Geometry: final body of the model. Coordinates: model frame, mm. A direction names the side the tool comes from. Round coordinates to 2 decimals unless told otherwise and drop trailing zeros. Loops run counter-clockwise (first coordinate to the right, second up) from the corner with the lowest first, then second, coordinate; pieces in that order, holes last. Notation, with made-up numbers: M -14,28.5 L 8,28.5 A30 ccw 8,64.5 Z; hole C 73,23 d4. An arc over 180 degrees is marked long. Write each question's results on one line, items separated by ' | '.
```python
from build123d import *

# Parameters (mm, degrees)
SZKIC1_W                       = 322
SZKIC1_H                       = 170
DODANIE_WYCI_GNI_CIE1_DEPTH    = 15
SZKIC2_R                       = 2
WYTNIJ_WYCI_GNI_CIE2_DEPTH     = 17.75
SZYK_LINIOWY1_COUNT            = 2
SZYK_LINIOWY1_PITCH            = 69.6
SZYK_LINIOWY1_COUNT_DIR2       = 2
SZYK_LINIOWY1_PITCH_DIR2       = 69.6
SZKIC5_R                       = 37.5
WYTNIJ_WYCI_GNI_CIE3_DEPTH     = 2
SZKIC7_R                       = 18.5
WYTNIJ_WYCI_GNI_CIE4_DEPTH     = 17.75
SZKIC10_R                      = 4
WYTNIJ_WYCI_GNI_CIE7_DEPTH     = 16
SZYK_LINIOWY3_COUNT            = 2
SZYK_LINIOWY3_PITCH            = 79
SZYK_LINIOWY2_COUNT            = 2
SZYK_LINIOWY2_PITCH            = 228
SZYK_LINIOWY2_COPY_1_SKETCH_R  = 2
SZYK_LINIOWY2_COPY_1_DEPTH     = 17.75
SZYK_LINIOWY2_COPY_2_SKETCH_R  = 2
SZYK_LINIOWY2_COPY_2_DEPTH     = 17.75
SZYK_LINIOWY2_COPY_3_SKETCH_R  = 2
SZYK_LINIOWY2_COPY_3_DEPTH     = 17.75
SZYK_LINIOWY2_COPY_4_SKETCH_R  = 4
SZYK_LINIOWY2_COPY_4_DEPTH     = 16
OTW_R_GWINTOWANY_M8X1_01_D     = 7
OTW_R_GWINTOWANY_M8X1_01_DEPTH = 21
OTW_R_GWINTOWANY_M8X1_01_TIP   = 2.103012167


with BuildPart() as part:
    # Szkic1 → Dodanie-wyci_gni_cie1 (new body)
    with BuildSketch(Plane.XY):
        Rectangle(SZKIC1_W, SZKIC1_H)
    extrude(amount=DODANIE_WYCI_GNI_CIE1_DEPTH)

    # Szkic2 → Wytnij-wyci_gni_cie2 (cut)
    with BuildSketch(Plane.XY.offset(15)):
        with Locations((-148.8, -71.87)):
            Circle(SZKIC2_R)
    wytnij_wyci_gni_cie2 = extrude(amount=-WYTNIJ_WYCI_GNI_CIE2_DEPTH, mode=Mode.SUBTRACT)

    # Szyk liniowy1: Wytnij-wyci_gni_cie2 2 × 2
    with Locations(*[(i * SZYK_LINIOWY1_PITCH, j * SZYK_LINIOWY1_PITCH_DIR2, 0) for i in range(SZYK_LINIOWY1_COUNT) for j in range(SZYK_LINIOWY1_COUNT_DIR2) if (i, j) != (0, 0)]):
        add(wytnij_wyci_gni_cie2, mode=Mode.SUBTRACT)

    # Szkic5 → Wytnij-wyci_gni_cie3 (cut)
    with BuildSketch(Plane(origin=(0, 0, 0), x_dir=(-1, 0, 0), z_dir=(0, 0, -1))):
        with Locations((114, -37.07)):
            Circle(SZKIC5_R)
    wytnij_wyci_gni_cie3 = extrude(amount=-WYTNIJ_WYCI_GNI_CIE3_DEPTH, mode=Mode.SUBTRACT)

    # Szkic7 → Wytnij-wyci_gni_cie4 (cut)
    with BuildSketch(Plane(origin=(0, 0, 2), x_dir=(-1, 0, 0), z_dir=(0, 0, -1))):
        with Locations((114, -37.07)):
            Circle(SZKIC7_R)
    wytnij_wyci_gni_cie4 = extrude(amount=-WYTNIJ_WYCI_GNI_CIE4_DEPTH, mode=Mode.SUBTRACT)

    # Szkic10 → Wytnij-wyci_gni_cie7 (cut, through all)
    with BuildSketch(Plane.XY.offset(15)):
        with Locations((-153.5, 42)):
            Circle(SZKIC10_R)
        with Locations((-153.5, 22)):
            Circle(SZKIC10_R)
    wytnij_wyci_gni_cie7 = extrude(amount=-WYTNIJ_WYCI_GNI_CIE7_DEPTH, mode=Mode.SUBTRACT)

    # Szyk liniowy3: Wytnij-wyci_gni_cie7 ×2
    with Locations(*[(i * SZYK_LINIOWY3_PITCH, 0, 0) for i in range(1, SZYK_LINIOWY3_COUNT)]):
        add(wytnij_wyci_gni_cie7, mode=Mode.SUBTRACT)

    # Szyk liniowy2: Wytnij-wyci_gni_cie2, Wytnij-wyci_gni_cie3, Wytnij-wyci_gni_cie4, Wytnij-wyci_gni_cie7 ×2
    with Locations(*[(i * SZYK_LINIOWY2_PITCH, 0, 0) for i in range(1, SZYK_LINIOWY2_COUNT)]):
        add(wytnij_wyci_gni_cie2, mode=Mode.SUBTRACT)
        add(wytnij_wyci_gni_cie3, mode=Mode.SUBTRACT)
        add(wytnij_wyci_gni_cie4, mode=Mode.SUBTRACT)
        add(wytnij_wyci_gni_cie7, mode=Mode.SUBTRACT)

    # Szyk liniowy2 copy 1 sketch → Szyk liniowy2 copy 1 (cut)
    with BuildSketch(Plane(origin=(228, 69.6, 15), x_dir=(1, 0, 0), z_dir=(0, 0, 1))):
        with Locations((-148.8, -71.87)):
            Circle(SZYK_LINIOWY2_COPY_1_SKETCH_R)
    extrude(amount=-SZYK_LINIOWY2_COPY_1_DEPTH, mode=Mode.SUBTRACT)

    # Szyk liniowy2 copy 2 sketch → Szyk liniowy2 copy 2 (cut)
    with BuildSketch(Plane(origin=(297.6, 0, 15), x_dir=(1, 0, 0), z_dir=(0, 0, 1))):
        with Locations((-148.8, -71.87)):
            Circle(SZYK_LINIOWY2_COPY_2_SKETCH_R)
    extrude(amount=-SZYK_LINIOWY2_COPY_2_DEPTH, mode=Mode.SUBTRACT)

    # Szyk liniowy2 copy 3 sketch → Szyk liniowy2 copy 3 (cut)
    with BuildSketch(Plane(origin=(297.6, 69.6, 15), x_dir=(1, 0, 0), z_dir=(0, 0, 1))):
        with Locations((-148.8, -71.87)):
            Circle(SZYK_LINIOWY2_COPY_3_SKETCH_R)
    extrude(amount=-SZYK_LINIOWY2_COPY_3_DEPTH, mode=Mode.SUBTRACT)

    # Szyk liniowy2 copy 4 sketch → Szyk liniowy2 copy 4 (cut, through all)
    with BuildSketch(Plane(origin=(307, 0, 15), x_dir=(1, 0, 0), z_dir=(0, 0, 1))):
        with Locations((-153.5, 42)):
            Circle(SZYK_LINIOWY2_COPY_4_SKETCH_R)
        with Locations((-153.5, 22)):
            Circle(SZYK_LINIOWY2_COPY_4_SKETCH_R)
    extrude(amount=-SZYK_LINIOWY2_COPY_4_DEPTH, mode=Mode.SUBTRACT)

    # Otw_r gwintowany M8x1.01
    with Locations(Plane(origin=(0, 85, 0), x_dir=(1, 0, 0), z_dir=(0, 1, 0))):
        with Locations((-152.5, -6.5), (-75.5, -6.5), (75.5, -6.5), (152.5, -6.5)):
            Hole(OTW_R_GWINTOWANY_M8X1_01_D / 2, depth=OTW_R_GWINTOWANY_M8X1_01_DEPTH)
            with Locations((0, 0, -(OTW_R_GWINTOWANY_M8X1_01_DEPTH + OTW_R_GWINTOWANY_M8X1_01_TIP / 2))):  # 118° drill point
                Cone(0, OTW_R_GWINTOWANY_M8X1_01_D / 2, OTW_R_GWINTOWANY_M8X1_01_TIP, mode=Mode.SUBTRACT)


solid = part.part
```
1. Section A-A (y = 42). Output: boundary loops of the cut face in (x, z).
Answer key:
outline: M -161,0 L -157.5,0 L -157.5,15 L -161,15 Z; M -149.5,0 L -78.5,0 L -78.5,15 L -149.5,15 Z; M -70.5,0 L 70.5,0 L 70.5,15 L -70.5,15 Z; M 78.5,0 L 149.5,0 L 149.5,15 L 78.5,15 Z; M 157.5,0 L 161,0 L 161,15 L 157.5,15 Z
2. Draft query along Z for faces 4 (the face through (79.36, -51.43, 0.99)), 5 (the face through (72.267, 74.353, 7.841)), 6 (the face through (106, -20, 2)). Return one class per face: pulls with the +Z half, pulls with the -Z half, needs draft (parallel to the pull), parting line crosses it, or undercut.
Answer key:
face 4: needs draft | face 5: undercut | face 6: pulls with the -Z half
3. Pin query (flat end, axial travel): P1, Ø4, axis at x = -152.5, z = 6.5, coming from the +Y side; P2, Ø4.5, axis at x = -79.2, y = -2.27, coming from the +Z side; P3, Ø4, axis at x = 110.5, y = -22.5, coming from the -Z side; P4, Ø1, axis at x = 93.5, y = -40.5, coming from the -Z side. Return the tip coordinate at first contact, or that it passes through.
Answer key:
P1: stops at y = 63.1 | P2: stops at z = 15 | P3: passes through | P4: stops at z = 2
4. Access query for faces 1 (the face through (-148.64, -51.43, 0.99)), 2 (the face through (149.16, 74.35, 5.45)), 3 (the face through (-2, 1, 0)). Directions: +Z, -Z, +X, -X, +Y, -Y. A direction counts if a zero-diameter tool reaches every point of the face in a straight line with its end or side. Return the directions, or none.
Answer key:
face 1: -Z | face 2: +Y | face 3: -Z, +X, -X, +Y, -Y
5. Ray query, probe 1 along Y at (x, z) = (-153.5, 11); probe 2 along Y at (x, z) = (114, 12.25); probe 3 along X at (y, z) = (-2.27, 6.25). Return the intervals inside material, ascending.
Answer key:
probe 1: y = -85 to 18, 26 to 38, 46 to 85 | probe 2: y = -85 to -55.57, -18.57 to 85 | probe 3: x = -161 to -150.8, -146.8 to -81.2, -77.2 to 77.2, 81.2 to 146.8, 150.8 to 161
6. Section B-B (z = 12.25). Count the separate pieces of the cut face and the enclosed holes in it, then the cut area to 3 significant figures.
Answer key:
separate pieces: 1 | enclosed holes: 18 | area: 52,100 mm²
